The model under review builds one solid part; all positions refer to its coordinate system, in mm. A direction names the side the tool comes from. Coordinates: 2 decimals unless noted, no trailing zeros. Loops run counter-clockwise (first coordinate to the right, second up) from the corner with the lowest first, then second, coordinate; pieces in that order, holes last. Notation, with made-up numbers: M -8.75,66 L 39.25,66 A34 cw 39.25,101 Z; hole C 59,20.25 d5. An arc over 180 degrees is marked long. Use CSV: the item, a comma, the result in double quotes. Start each with the question number.
1. Add section C-C, the plane x = 0.5. Write out the cut boundary in (y, z).
2. Add section A-A, the plane y = -0.5. Write out the cut boundary in (x, z), then the cut area to 3 significant figures.
3. Tool access review of faces 5 (the flat face through (1, -1.524, 1)), 6 (the flat face through (0, -2, 1.524)): name each direction out of +Z, -Z, +X, -X, +Y, -Y from which nothing blocks a thin tool from reaching the whole face with its end or side.
4. Add section B-B, the plane z = 1.3. Write out the cut boundary in (x, y), then the cut area to 3 significant figures.
5. For L1, parallel to X at y = -1, z = 0.4; L2, parallel to X at y = -1.25, z = 0.9; L3, parallel to Y at x = 0.5, z = 0.55, list the stretches that pass through material, from the lowest coordinate up.
6. Draft analysis for pull direction Y (two halves, no side actions). For faces 1 (the flat face through (0, -1, 1)), 2 (the cylindrical face through (-0.45, 2.5, 0.75)), 3 (the flat face through (1.524, -1, 1)), 4 (the cylindrical face through (-0.99, -3.025, 0.751)), state which applies: +Y half, -Y half, draft (parallel to the pull), parting line (faces both ways), or undercut.
7. Add section D-D, the plane x = 4. Write out the cut boundary in (y, z), then the cut area to 3 significant figures.
from build123d import *

# Parameters (mm, degrees)
SKETCH1_W           = 1.524
SKETCH1_H           = 1.524
BOSS_EXTRUDE1_DEPTH = 1.524


with BuildPart() as part:
    # Sketch1 → Boss-Extrude1 (new body)
    with BuildSketch(Plane.XY):
        with BuildLine():
            ThreePointArc((-4.813018271, 1.647414383), (-6.381436297, -1.405112195), (-3.535820464, -3.323529288))
            ThreePointArc((-3.535820464, -3.323529288), (-0.953914357, -3.028591374), (1.524, -3.811641797))
            ThreePointArc((1.524, -3.811641797), (6.486387953, -2.185545764), (3.86325293, 2.329832974))
            ThreePointArc((3.86325293, 2.329832974), (-0.514779052, 2.495866349), (-4.813018271, 1.647414383))
        make_face()
        with Locations((0.762, -0.762)):
            Rectangle(SKETCH1_W, SKETCH1_H, mode=Mode.SUBTRACT)
    extrude(amount=BOSS_EXTRUDE1_DEPTH)


solid = part.part
Computed:
1,outline,"M -3.35,0 L -1.52,0 L -1.52,1.52 L -3.35,1.52 Z; M 0,0 L 2.55,0 L 2.55,1.52 L 0,1.52 Z"
2,outline,"M -6.45,0 L 0,0 L 0,1.52 L -6.45,1.52 Z; M 1.52,0 L 6.67,0 L 6.67,1.52 L 1.52,1.52 Z"
2,area,"17.7 mm^2"
3,face 5,"+Z, -Z"
3,face 6,"+Z, +X, -X, +Y, -Y"
4,outline,"M -4.81,1.65 A2.58 ccw -3.54,-3.32 A6.24 cw 1.52,-3.81 A3.36 ccw long 3.86,2.33 A18.86 ccw Z; hole M 0,-1.52 L 1.52,-1.52 L 1.52,0 L 0,0 Z"
4,area,"68.2 mm^2"
5,L1,"x = -6.45 to 0, 1.52 to 6.71"
5,L2,"x = -6.42 to 0, 1.52 to 6.7"
5,L3,"y = -3.35 to -1.52, 0 to 2.55"
6,face 1,"undercut"
6,face 2,"+Y half"
6,face 3,"undercut"
6,face 4,"-Y half"
7,outline,"M -4.29,0 L 2.31,0 L 2.31,1.52 L -4.29,1.52 Z"
7,area,"10.0 mm^2"
